Input: part model. Units: mm. Frame: model coordinates. A direction names the side the tool comes from. Round coordinates to 2 decimals unless told otherwise and drop trailing zeros. Loops run counter-clockwise (first coordinate to the right, second up) from the corner with the lowest first, then second, coordinate; pieces in that order, holes last. Notation, with made-up numbers: (75, 60) - (128, 60) arc R26 ccw to (128, 88) - close; hole circle Ø4 at (84, 60.5). An arc over 180 degrees is marked (long way). One line per question, with ' | ' between items. Start each with the question number.
from build123d import *

# Parameters (mm, degrees)
BOSS_EXTRUDE1_DEPTH = 127
CUT_EXTRUDE1_DEPTH  = 88.9
CUT_EXTRUDE2_DEPTH  = 1.27
CUT_EXTRUDE3_DEPTH  = 6.35
SKETCH6_R           = 1.27
BOSS_EXTRUDE2_DEPTH = 3.81


with BuildPart() as part:
    # Sketch1 → Boss-Extrude1 (new body)
    with BuildSketch(Plane(origin=(0, 0, 0), x_dir=(1, 0, 0), z_dir=(0, 1, 0))):
        with BuildLine():
            Line((0, 0), (42.739614803, 0))
            Line((42.739614803, 0), (42.739614803, -42.739614803))
            ThreePointArc((42.739614803, -42.739614803), (21.369807402, -47.941054373), (0, -42.739614803))
            Line((0, -42.739614803), (0, 0))
        make_face()
    extrude(amount=BOSS_EXTRUDE1_DEPTH)

    # Sketch2 → Cut-Extrude1 (cut)
    with BuildSketch(Plane.XY.offset(127)):
        with BuildLine():
            Line((13.881687598, 110.608783011), (28.857927206, 110.608783011))
            ThreePointArc((28.857927206, 110.608783011), (34.246080878, 108.376936683), (36.477927206, 102.988783011))
            Line((36.477927206, 102.988783011), (36.477927206, 68.734309223))
            Line((36.477927206, 68.734309223), (6.261687598, 68.734309223))
            Line((6.261687598, 68.734309223), (6.261687598, 102.988783011))
            ThreePointArc((6.261687598, 102.988783011), (8.493533925, 108.376936683), (13.881687598, 110.608783011))
        make_face()
    extrude(amount=-CUT_EXTRUDE1_DEPTH, mode=Mode.SUBTRACT)

    # Sketch4 → Cut-Extrude2 (cut)
    with BuildSketch(Plane(origin=(0, 68.734309223, 0), x_dir=(1, 0, 0), z_dir=(0, 1, 0))):
        with BuildLine():
            Line((18.101107041, -45.607119247), (24.638507762, -45.607119247))
            ThreePointArc((24.638507762, -45.607119247), (25.019507762, -45.226119247), (24.638507762, -44.845119247))
            Line((24.638507762, -44.845119247), (18.101107041, -44.845119247))
            ThreePointArc((18.101107041, -44.845119247), (17.720107041, -45.226119247), (18.101107041, -45.607119247))
        make_face()
        with BuildLine():
            Line((8.722196959, -45.607119247), (15.25959768, -45.607119247))
            ThreePointArc((15.25959768, -45.607119247), (15.64059768, -45.226119247), (15.25959768, -44.845119247))
            Line((15.25959768, -44.845119247), (8.722196959, -44.845119247))
            ThreePointArc((8.722196959, -44.845119247), (8.341196959, -45.226119247), (8.722196959, -45.607119247))
        make_face()
        with BuildLine():
            Line((8.722196959, -42.559119247), (15.25959768, -42.559119247))
            ThreePointArc((15.25959768, -42.559119247), (15.64059768, -42.178119247), (15.25959768, -41.797119247))
            Line((15.25959768, -41.797119247), (8.722196959, -41.797119247))
            ThreePointArc((8.722196959, -41.797119247), (8.341196959, -42.178119247), (8.722196959, -42.559119247))
        make_face()
        with BuildLine():
            Line((8.722196959, -44.083119247), (15.25959768, -44.083119247))
            ThreePointArc((15.25959768, -44.083119247), (15.64059768, -43.702119247), (15.25959768, -43.321119247))
            Line((15.25959768, -43.321119247), (8.722196959, -43.321119247))
            ThreePointArc((8.722196959, -43.321119247), (8.341196959, -43.702119247), (8.722196959, -44.083119247))
        make_face()
        with BuildLine():
            Line((18.101107041, -44.083119247), (24.638507762, -44.083119247))
            ThreePointArc((24.638507762, -44.083119247), (25.019507762, -43.702119247), (24.638507762, -43.321119247))
            Line((24.638507762, -43.321119247), (18.101107041, -43.321119247))
            ThreePointArc((18.101107041, -43.321119247), (17.720107041, -43.702119247), (18.101107041, -44.083119247))
        make_face()
        with BuildLine():
            Line((18.101107041, -42.559119247), (24.638507762, -42.559119247))
            ThreePointArc((24.638507762, -42.559119247), (25.019507762, -42.178119247), (24.638507762, -41.797119247))
            Line((24.638507762, -41.797119247), (18.101107041, -41.797119247))
            ThreePointArc((18.101107041, -41.797119247), (17.720107041, -42.178119247), (18.101107041, -42.559119247))
        make_face()
        with BuildLine():
            Line((18.101107041, -41.035119247), (24.638507762, -41.035119247))
            ThreePointArc((24.638507762, -41.035119247), (25.019507762, -40.654119247), (24.638507762, -40.273119247))
            Line((24.638507762, -40.273119247), (18.101107041, -40.273119247))
            ThreePointArc((18.101107041, -40.273119247), (17.720107041, -40.654119247), (18.101107041, -41.035119247))
        make_face()
        with BuildLine():
            Line((18.101107041, -39.511119247), (24.638507762, -39.511119247))
            ThreePointArc((24.638507762, -39.511119247), (25.019507762, -39.130119247), (24.638507762, -38.749119247))
            Line((24.638507762, -38.749119247), (18.101107041, -38.749119247))
            ThreePointArc((18.101107041, -38.749119247), (17.720107041, -39.130119247), (18.101107041, -39.511119247))
        make_face()
        with BuildLine():
            Line((8.722196959, -41.035119247), (15.25959768, -41.035119247))
            ThreePointArc((15.25959768, -41.035119247), (15.64059768, -40.654119247), (15.25959768, -40.273119247))
            Line((15.25959768, -40.273119247), (8.722196959, -40.273119247))
            ThreePointArc((8.722196959, -40.273119247), (8.341196959, -40.654119247), (8.722196959, -41.035119247))
        make_face()
        with BuildLine():
            Line((8.722196959, -39.511119247), (15.25959768, -39.511119247))
            ThreePointArc((15.25959768, -39.511119247), (15.64059768, -39.130119247), (15.25959768, -38.749119247))
            Line((15.25959768, -38.749119247), (8.722196959, -38.749119247))
            ThreePointArc((8.722196959, -38.749119247), (8.341196959, -39.130119247), (8.722196959, -39.511119247))
        make_face()
        with BuildLine():
            Line((27.480017123, -44.083119247), (34.017417844, -44.083119247))
            ThreePointArc((34.017417844, -44.083119247), (34.398417844, -43.702119247), (34.017417844, -43.321119247))
            Line((34.017417844, -43.321119247), (27.480017123, -43.321119247))
            ThreePointArc((27.480017123, -43.321119247), (27.099017123, -43.702119247), (27.480017123, -44.083119247))
        make_face()
        with BuildLine():
            Line((27.480017123, -42.559119247), (34.017417844, -42.559119247))
            ThreePointArc((34.017417844, -42.559119247), (34.398417844, -42.178119247), (34.017417844, -41.797119247))
            Line((34.017417844, -41.797119247), (27.480017123, -41.797119247))
            ThreePointArc((27.480017123, -41.797119247), (27.099017123, -42.178119247), (27.480017123, -42.559119247))
        make_face()
        with BuildLine():
            Line((27.480017123, -41.035119247), (34.017417844, -41.035119247))
            ThreePointArc((34.017417844, -41.035119247), (34.398417844, -40.654119247), (34.017417844, -40.273119247))
            Line((34.017417844, -40.273119247), (27.480017123, -40.273119247))
            ThreePointArc((27.480017123, -40.273119247), (27.099017123, -40.654119247), (27.480017123, -41.035119247))
        make_face()
        with BuildLine():
            Line((27.480017123, -39.511119247), (34.017417844, -39.511119247))
            ThreePointArc((34.017417844, -39.511119247), (34.398417844, -39.130119247), (34.017417844, -38.749119247))
            Line((34.017417844, -38.749119247), (27.480017123, -38.749119247))
            ThreePointArc((27.480017123, -38.749119247), (27.099017123, -39.130119247), (27.480017123, -39.511119247))
        make_face()
        with BuildLine():
            ThreePointArc((27.480017123, -44.845119247), (27.099017123, -45.226119247), (27.480017123, -45.607119247))
            Line((27.480017123, -45.607119247), (34.017417844, -45.607119247))
            ThreePointArc((34.017417844, -45.607119247), (34.398417844, -45.226119247), (34.017417844, -44.845119247))
            Line((34.017417844, -44.845119247), (27.480017123, -44.845119247))
        make_face()
    extrude(amount=-CUT_EXTRUDE2_DEPTH, mode=Mode.SUBTRACT)

    # Sketch5 → Cut-Extrude3 (cut)
    with BuildSketch(Plane(origin=(0, 127, 0), x_dir=(1, 0, 0), z_dir=(0, 1, 0))):
        with BuildLine():
            ThreePointArc((27.058825704, -21.369807402), (21.369807402, -15.680789099), (15.680789099, -21.369807402))
            Line((15.680789099, -21.369807402), (27.058825704, -21.369807402))
        make_face()
        with BuildLine():
            Line((27.058825704, -21.369807402), (15.680789099, -21.369807402))
            ThreePointArc((15.680789099, -21.369807402), (21.369807402, -27.058825704), (27.058825704, -21.369807402))
        make_face()
    extrude(amount=-CUT_EXTRUDE3_DEPTH, mode=Mode.SUBTRACT)

    # Sketch6 → Boss-Extrude2 (add)
    with BuildSketch(Plane.XY.offset(38.1)):
        with Locations(Location((17.026937254, 96.316061715, 0), (0, 0, 180))):
            Circle(SKETCH6_R)
        with Locations(Location((25.712677549, 96.316061715, 0), (0, 0, 180))):
            Circle(SKETCH6_R)
    extrude(amount=BOSS_EXTRUDE2_DEPTH)

    # Sketch8 → Revolve1 (revolve)
    with BuildSketch(Plane.YZ.offset(17.026937254), mode=Mode.PRIVATE) as revolve1_sk:
        Polygon((92.462776609, 42.625909045), (92.462776609, 43.341818089), (98.173073883, 44.293534302), (98.173073883, 42.739614803), align=None)
    revolve1 = revolve(revolve1_sk.sketch.rotate(Axis((17.026937254, 92.462776609, 42.625909045), (0, 0.9998018069764348, 0.01990845967561906)), 180), axis=Axis((17.026937254, 92.462776609, 42.625909045), (0, 0.9998018069764348, 0.01990845967561906)))

    # Mirror1: Revolve1 across plane
    add(revolve1.mirror(Plane.ZY.offset(-21.369807402)))


solid = part.part
(1) Reachability of faces 1 (the face through (22, 0, 24)), 2 (the face through (6.262, 86, 42)), 3 (the face through (16.977, 95.358, 43.823)), 4 (the face through (18.745, 123.869, 16.323)) from +Z, -Z, +X, -X, +Y, -Y: full face, straight path, thin tool, end or side. Return the list, or none.
(2) Section C-C, the plane y = 64. Output: boundary loops of the cut face in (x, z).
(3) Pin query (flat end, axial travel): P1, Ø12, axis at x = 36.5, y = 26, coming from the +Z side; P2, Ø0.6, axis at x = 31.5, y = 68, coming from the -Z side; P3, Ø1.4, axis at x = 20, y = 68, coming from the +Z side; P4, Ø0.6, axis at x = 13, y = 68.5, coming from the +Z side. Return the tip coordinate at first contact, or that it passes through.
(4) Section A-A, the plane y = 100. Output: boundary loops of the cut face in (x, z).
(5) Line query: line 1 along Y through (x, z) = (24.5, 45.5); line 2 along Y through (x, z) = (16.5, 22); line 3 along Z through (x, y) = (29, 116.5). Output: solid intervals per line, ascending. Write a range as from..to.
(6) Section B-B, the plane x = 5. Output: boundary loops of the cut face in (y, z), plus the area to 3 significant figures.
(7) Pull-direction query (X, two-part tool) for faces 5 (the face through (22, 90, 38.1)), 6 (the face through (21.68, 48.5, 47.94)), 7 (the face through (0, 63, 22)), 8 (the face through (21, 63, 0)); classes: released by +X, released by -X, zero draft, split by the parting line, or undercut.
Derived:
1) face 1: +Z, -Z, +X, -X, -Y | face 2: +Z | face 3: none | face 4: +Y
2) outline: (0, 0) - (42.74, 0) - (42.74, 42.74) arc R46.5 ccw to (0, 42.74) - close
3) P1: stops at z = 47.04 | P2: stops at z = 0 | P3: stops at z = 47.94 | P4: stops at z = 47.24
4) outline: (0, 0) - (42.74, 0) - (42.74, 42.74) arc R46.5 ccw to (36.48, 45.42) - (36.48, 38.1) - (6.26, 38.1) - (6.26, 45.42) arc R46.5 ccw to (0, 42.74) - close
5) line 1: y = 0..67.46, 110.61..127 | line 2: y = 0..120.65 | line 3: z = 0..47.31
6) outline: (0, 0) - (127, 0) - (127, 44.96) - (0, 44.96) - close | area: 5,710 mm²
7) face 5: undercut | face 6: split by the parting line | face 7: released by -X | face 8: zero draft
